Read the model definition and answer for the solid it produces. Units are mm, in the model's axes. A direction names the side the tool comes from. Round coordinates to 2 decimals unless told otherwise and drop trailing zeros. Loops run counter-clockwise (first coordinate to the right, second up) from the corner with the lowest first, then second, coordinate; pieces in that order, holes last. Notation, with made-up numbers: M -22,49 L 15,49 A24 cw 15,82 Z; hole C 54.25,-17 d4. An arc over 180 degrees is marked long. Write each question's results on one line, items separated by ' | '.
from build123d import *

# Parameters (mm, degrees)
F1_DEPTH = 330.2
F3_DEPTH = 50.8
F5_DEPTH = 50.8


with BuildPart() as f1:
    # F0 (on Front) → F1 (new body, symmetric)
    with BuildSketch(Plane.XZ):
        Polygon((-584.2, 457.2), (-584.2, 0), (-558.8, 0), (-558.8, 431.8), (558.8, 431.8), (558.8, 0), (584.2, 0), (584.2, 457.2), align=None)
    extrude(amount=F1_DEPTH, both=True)

    # F2 (on face) → F3 (join)
    with BuildSketch(Plane(origin=(0, 330.2, 0), x_dir=(-1, 0, 0), z_dir=(0, 1, 0))):
        Polygon((-558.8, 431.8), (-558.8, 0), (-508, 0), (-508, 381), (508, 381), (508, 0), (558.8, 0), (558.8, 431.8), align=None)
    extrude(amount=-F3_DEPTH)

    # F4 (on face) → F5 (join)
    with BuildSketch(Plane.XZ.offset(330.2)):
        Polygon((-584.2, 457.2), (-584.2, 0), (-508, 0), (-508, 381), (508, 381), (508, 0), (584.2, 0), (584.2, 457.2), align=None)
    extrude(amount=-F5_DEPTH)


solid = f1.part
Item 1: The mould has two halves that part along X. Classify faces 1 (the face through (-8, -330.2, 384)), 2 (the face through (-584.2, -5, 232)), 3 (the face through (3, 279.4, 393)), 4 (the face through (508, -305, 193)): pulls with the +X half, pulls with the -X half, needs draft (parallel to the pull), parting line crosses it, or undercut.
Outcome:
face 1: needs draft | face 2: pulls with the -X half | face 3: undercut | face 4: undercut
Item 2: The part is cut by section D-D (y = -20). Determine the outline of the cut face in (x, z).
Outcome:
outline: M -584.2,0 L -558.8,0 L -558.8,431.8 L 558.8,431.8 L 558.8,0 L 584.2,0 L 584.2,457.2 L -584.2,457.2 Z
Item 3: The part is cut by section B-B (z = 261). Determine the outline of the cut face in (x, y), plus the area to 3 significant figures.
Outcome:
outline: M -584.2,-330.2 L -508,-330.2 L -508,-279.4 L -558.8,-279.4 L -558.8,279.4 L -508,279.4 L -508,330.2 L -584.2,330.2 Z; M 508,-330.2 L 584.2,-330.2 L 584.2,330.2 L 508,330.2 L 508,279.4 L 558.8,279.4 L 558.8,-279.4 L 508,-279.4 Z | area: 43,900 mm2
Item 4: Straight lines are drawn through the part: line 1 (Y direction, x = -536, z = 92.5); line 2 (X direction, y = 231, z = 207); line 3 (X direction, y = -296, z = 374). For each, find the intervals that lie inside material, in ascending order.
Outcome:
line 1: y = -330.2 to -279.4, 279.4 to 330.2 | line 2: x = -584.2 to -558.8, 558.8 to 584.2 | line 3: x = -584.2 to -508, 508 to 584.2
Item 5: For faces 5 (the face through (564, 5, 0)), 6 (the face through (-8, -4, 431.8)), 7 (the face through (-508, -305, 188)), determine the directions among +Z, -Z, +X, -X, +Y, -Y from which every point of the face is accessible in a straight line to the end or side of a thin tool.
Outcome:
face 5: -Z, +X, -X, +Y, -Y | face 6: -Z | face 7: -Z, +Y, -Y
Item 6: The part is cut by section C-C (x = -408). Determine the outline of the cut face in (y, z), plus the area to 3 significant figures.
Outcome:
outline: M -330.2,381 L -279.4,381 L -279.4,431.8 L 279.4,431.8 L 279.4,381 L 330.2,381 L 330.2,457.2 L -330.2,457.2 Z | area: 21,900 mm2
Item 7: The part is cut by section A-A (z = 397). Determine the outline of the cut face in (x, y).
Outcome:
outline: M -584.2,-330.2 L 584.2,-330.2 L 584.2,330.2 L -584.2,330.2 Z; hole M -558.8,-279.4 L 558.8,-279.4 L 558.8,279.4 L -558.8,279.4 Z
